from build123d import *

# Parameters (mm, degrees)
SKETCH2_OUTSIDE_W  = 32.552
SKETCH2_OUTSIDE_H  = 32.553
CUT_EXTRUDE1_DEPTH = 25.2984
CHAMFER1_SIZE      = 0.508
FILLET1_R          = 0.635


with BuildPart() as part:
    # Sketch1 → Revolve1 (revolve)
    with BuildSketch(Plane(origin=(0, 0, 0), x_dir=(0, 0, -1), z_dir=(1, 0, 0))):
        Polygon((0, 0), (0, 6.35), (7.9502, 6.35), (7.9502, 7.62), (33.2486, 7.62), (33.2486, 7.9375), (61.9252, 7.9375), (61.9252, 6.35), (69.8754, 6.35), (69.8754, 0), align=None)
    revolve(axis=Axis((0, 0, 0), (0, 0, 1)))

    # Sketch2 outside → Cut-Extrude1 (cut)
    with BuildSketch(Plane.XY.offset(-7.9502)):
        with Locations((0, 0.0005)):
            Rectangle(SKETCH2_OUTSIDE_W, SKETCH2_OUTSIDE_H)
        Polygon((3.696970073, 6.40334), (-3.696970073, 6.40334), (-7.393940145, 0), (-3.696970073, -6.40334), (3.696970073, -6.40334), (7.393940145, 0), align=None, mode=Mode.SUBTRACT)
    extrude(amount=-CUT_EXTRUDE1_DEPTH, mode=Mode.SUBTRACT)

    # Chamfer1
    chamfer1_edges = [part.edges().sort_by_distance(p)[0] for p in [
        (0, -6.35, 0),
        (0, -6.35, -69.8754),
    ]]
    chamfer(chamfer1_edges, length=CHAMFER1_SIZE)

    # Fillet1
    fillet1_edges = [part.edges().sort_by_distance(p)[0] for p in [
        (3.696970073, 6.40334, -20.5994),
        (-3.696970073, 6.40334, -20.5994),
        (-7.393940145, 0, -20.5994),
        (-3.696970073, -6.40334, -20.5994),
        (3.696970073, -6.40334, -20.5994),
        (7.393940145, 0, -20.5994),
    ]]
    fillet(fillet1_edges, radius=FILLET1_R)


solid = part.part
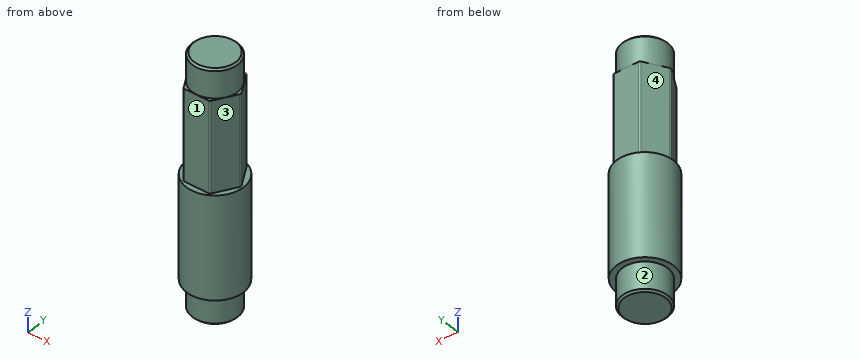
Check sheet for the modelled part. Datum: model origin and axes. Units: mm. Face numbers are marked on the shaded views. A direction names the side the tool comes from. Give positions to 0.01 mm unless a question says otherwise; leave off trailing zeros. Loops run counter-clockwise (first coordinate to the right, second up) from the corner with the lowest first, then second, coordinate; pieces in that order, holes last. Notation, with made-up numbers: M 69.25,77.5 L 77.25,77.5 A27 ccw 77.25,103.5 Z; hole C 46,23 d2. An arc over 180 degrees is marked long. Answer as a JSON object with one key per item and string values. Group by question number.
Q1. Cross-section at B-B on x = 0. Record the cut outline in (y, z).
Q2. Access from +Z, -Z, +X, -X, +Y, -Y to the whole of each face (thin tool, end or side, straight path). Record for the marked faces 1, 2, 3 and 4.
Q3. Go/stop test with flat-tipped pins: P1, Ø6, axis at y = 2, z = -37, coming from the +X side; P2, Ø7.5, axis at x = -0.5, z = -17.5, coming from the +Y side; P3, Ø5, axis at y = 2, z = -18, coming from the +X side; P4, Ø3, axis at x = -3.5, z = -38.5, coming from the +Y side. Record where each tip stops, or that it passes through.
Q4. Material ranges on line 1 along Y through (x, z) = (-1, -23.5); line 2 along Z through (x, y) = (6, 2.25); line 3 along Y through (x, z) = (1.75, -52.5), recorded low to high. Write a range as [from, to].
Q5. Cross-section at D-D on z = -50. Record the cut outline in (x, y) (1 decimal).
Q6. Cross-section at A-A on z = -25.5. Record the cut outline in (x, y) (1 decimal).
Q7. Cross-section at C-C on y = 7. Record the cut outline in (x, z).
Evaluation:
{
 "1": {"outline": "M -7.94,-61.93 L -6.35,-61.93 L -6.35,-69.37 L -5.84,-69.88 L 5.84,-69.88 L 6.35,-69.37 L 6.35,-61.93 L 7.94,-61.93 L 7.94,-33.25 L 6.4,-33.25 L 6.4,-7.95 L 6.35,-7.95 L 6.35,-0.51 L 5.84,0 L -5.84,0 L -6.35,-0.51 L -6.35,-7.95 L -6.4,-7.95 L -6.4,-33.25 L -7.94,-33.25 Z"},
 "2": {"face 1": "+Z, +X, -X, -Y", "face 2": "-Z", "face 3": "+Z, +X, -Y", "face 4": "+Z, -X, +Y"},
 "3": {"P1": "stops at x = 7.94", "P2": "stops at y = 6.4", "P3": "stops at x = 7.3", "P4": "stops at y = 7.68"},
 "4": {"line 1": "y = [-6.4, 6.4]", "line 2": "z = [-61.93, -7.95]", "line 3": "y = [-7.74, 7.74]"},
 "5": {"outline": "C 0,0 d15.9"},
 "6": {"outline": "M -7.2,-0.3 L -3.9,-6.1 A0.6 ccw -3.3,-6.4 L 3.3,-6.4 A0.6 ccw 3.9,-6.1 L 7.2,-0.3 A0.6 ccw 7.2,0.3 L 3.9,6.1 A0.6 ccw 3.3,6.4 L -3.3,6.4 A0.6 ccw -3.9,6.1 L -7.2,0.3 A0.6 ccw Z"},
 "7": {"outline": "M -3.74,-61.93 L 3.74,-61.93 L 3.74,-33.25 L -3.74,-33.25 Z"}
}
